from build123d import *

# Parameters (mm, degrees)
SKETCH1_W           = 30.1
SKETCH1_H           = 34.1
SKETCH1_W_2         = 26.1
SKETCH1_H_2         = 30.1
BOSS_EXTRUDE1_DEPTH = 5
SKETCH2_W           = 10.8
SKETCH2_H           = 2
SKETCH2_W_2         = 4.6
BOSS_EXTRUDE2_DEPTH = 8
SKETCH3_R           = 1.7
CUT_EXTRUDE1_DEPTH  = 25.108193628
SKETCH4_R           = 2.8
CUT_EXTRUDE2_DEPTH  = 3
SKETCH6_W           = 26.1
SKETCH6_H           = 20.05
SKETCH6_R           = 2.75
BOSS_EXTRUDE3_DEPTH = 5


with BuildPart() as part:
    # Sketch1 → Boss-Extrude1 (new body)
    # profile 1 of 2: a face of its own
    with BuildSketch(Plane(origin=(0, 0, 0), x_dir=(0, 0, -1), z_dir=(1, 0, 0))):
        Rectangle(SKETCH1_W, SKETCH1_H)
        Rectangle(SKETCH1_W_2, SKETCH1_H_2, mode=Mode.SUBTRACT)
    # profile 2 of 2: a face of its own
    with BuildSketch(Plane(origin=(0, 0, 0), x_dir=(0, 0, -1), z_dir=(1, 0, 0))):
        Rectangle(SKETCH1_W_2, SKETCH1_H_2)
    extrude(amount=BOSS_EXTRUDE1_DEPTH)

    # Sketch2 → Boss-Extrude2 (add)
    with BuildSketch(Plane(origin=(5, 0, 0), x_dir=(0, 0, -1), z_dir=(1, 0, 0))):
        with Locations((7.65, -16.05)):
            Rectangle(SKETCH2_W, SKETCH2_H)
        Polygon((13.05, 15.05), (13.05, -15.05), (13.05, -17.05), (15.05, -17.05), (15.05, 17.05), (13.05, 17.05), align=None)
        with Locations((6.15, 16.05)):
            Rectangle(SKETCH2_W_2, SKETCH2_H)
        with Locations((-6.15, 16.05)):
            Rectangle(SKETCH2_W_2, SKETCH2_H)
        Polygon((-13.05, -15.05), (-13.05, 15.05), (-13.05, 17.05), (-15.05, 17.05), (-15.05, -17.05), (2.25, -17.05), (2.25, -15.05), align=None)
    extrude(amount=BOSS_EXTRUDE2_DEPTH)

    # Sketch3 → Cut-Extrude1 (cut, through all)
    with BuildSketch(Plane(origin=(5, 0, 0), x_dir=(0, 0, -1), z_dir=(1, 0, 0))):
        with Locations((0, -10)):
            Circle(SKETCH3_R)
        Circle(SKETCH3_R)
        with Locations((0, 10)):
            Circle(SKETCH3_R)
    extrude(amount=-CUT_EXTRUDE1_DEPTH, mode=Mode.SUBTRACT)

    # Sketch4 → Cut-Extrude2 (cut)
    with BuildSketch(Plane(origin=(5, 0, 0), x_dir=(0, 0, -1), z_dir=(1, 0, 0))):
        with Locations((0, -10)):
            Circle(SKETCH4_R)
        Circle(SKETCH4_R)
        with Locations((0, 10)):
            Circle(SKETCH4_R)
    extrude(amount=-CUT_EXTRUDE2_DEPTH, mode=Mode.SUBTRACT)

    # Sketch6 → Boss-Extrude3 (add)
    with BuildSketch(Plane(origin=(5, 0, 0), x_dir=(0, 0, -1), z_dir=(1, 0, 0))):
        with Locations((0, -5.025)):
            Rectangle(SKETCH6_W, SKETCH6_H)
        Circle(SKETCH6_R, mode=Mode.SUBTRACT)
        with Locations((0, -10)):
            Circle(SKETCH6_R, mode=Mode.SUBTRACT)
    extrude(amount=BOSS_EXTRUDE3_DEPTH)


solid = part.part
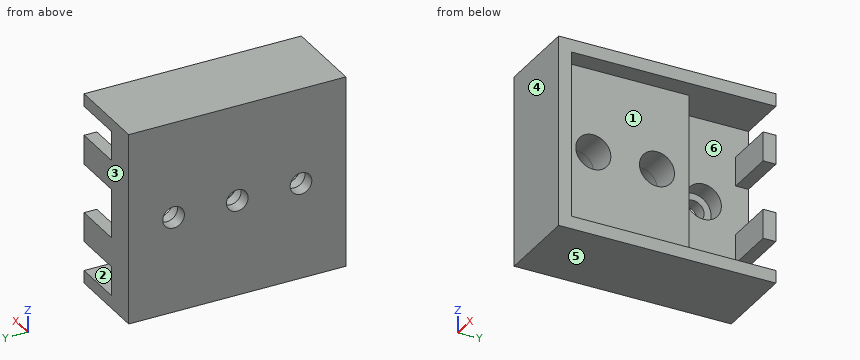
Verification items for the finished model (mm, model axes). Face numbers are marked on the shaded views. A direction names the side the tool comes from. Coordinates: 2 decimals unless noted, no trailing zeros. Order: outer loops, then holes, each group sorted by start corner. A loop starts at its lowest first (then second) coordinate and runs counter-clockwise, first axis right, second up. Notation, with made-up numbers: M 34.25,-36.5 L 53.25,-36.5 A13 ccw 53.25,-21.5 Z; hole C -6.75,43 d5. An arc over 180 degrees is marked long. One line per item, written item: value. Start each with the question number.
Item 1: Sectioned sample at D-D on z = -5. Record the cut outline in (x, y).
Item 2: Thickness scan on probe 1 along Y at (x, z) = (1.2, 0); probe 2 along Z at (x, y) = (8.25, 16.5); probe 3 along Y at (x, z) = (4.1, 0). Record the ranges inside material, lowest first.
Item 3: Mould release check, pull along Z, two halves, no side actions. Record for the marked faces 4, 5 and 6: pulls with the +Z half, pulls with the -Z half, needs draft (parallel to the pull), parting line crosses it, or undercut.
Item 4: Access from +Z, -Z, +X, -X, +Y, -Y to the whole of each face (thin tool, end or side, straight path). Record for the marked faces 1, 2 and 3.
Item 5: Depth check by flat-ended pin: P1, Ø1.7, axis at y = 0.5, z = 0, coming from the -X side; P2, Ø16, axis at y = -5.5, z = 4.5, coming from the +X side; P3, Ø4.5, axis at y = 10, z = 0, coming from the +X side. Enter the tip coordinate at first touch or a pass-through.
Item 6: Sectioned sample at C-C on x = 3. Record the cut outline in (y, z).
Item 7: Sectioned sample at A-A on x = 5.5. Record the cut outline in (y, z).
Item 8: Sectioned sample at B-B on y = 10. Record the cut outline in (x, z).
Calculated:
1. outline: M 0,-17.05 L 13,-17.05 L 13,-15.05 L 10,-15.05 L 10,5 L 5,5 L 5,15.05 L 13,15.05 L 13,17.05 L 0,17.05 Z
2. probe 1: -17.05 to -11.7, -8.3 to -1.7, 1.7 to 8.3, 11.7 to 17.05
2. probe 2: -15.05 to -13.05, -8.45 to -3.85, 3.85 to 8.45, 13.05 to 15.05
2. probe 3: -17.05 to -12.8, -7.2 to -2.8, 2.8 to 7.2, 12.8 to 17.05
3. face 4: needs draft
3. face 5: pulls with the -Z half
3. face 6: undercut
4. face 1: +X
4. face 2: +X, +Y
4. face 3: +Z, -Z, +X, -X, +Y
5. P1: through
5. P2: x = 10
5. P3: x = 2
6. outline: M -17.05,-15.05 L 17.05,-15.05 L 17.05,15.05 L -17.05,15.05 Z; hole C -10,0 d5.6; hole C 0,0 d5.6; hole C 10,0 d5.6
7. outline: M -17.05,-15.05 L 17.05,-15.05 L 17.05,-13.05 L 5,-13.05 L 5,13.05 L 17.05,13.05 L 17.05,15.05 L -17.05,15.05 Z; M 15.05,-8.45 L 17.05,-8.45 L 17.05,-3.85 L 15.05,-3.85 Z; M 15.05,3.85 L 17.05,3.85 L 17.05,8.45 L 15.05,8.45 Z; hole C -10,0 d5.5; hole C 0,0 d5.5
8. outline: M 0,-15.05 L 13,-15.05 L 13,-13.05 L 5,-13.05 L 5,-2.8 L 2,-2.8 L 2,-1.7 L 0,-1.7 Z; M 0,1.7 L 2,1.7 L 2,2.8 L 5,2.8 L 5,13.05 L 13,13.05 L 13,15.05 L 0,15.05 Z
